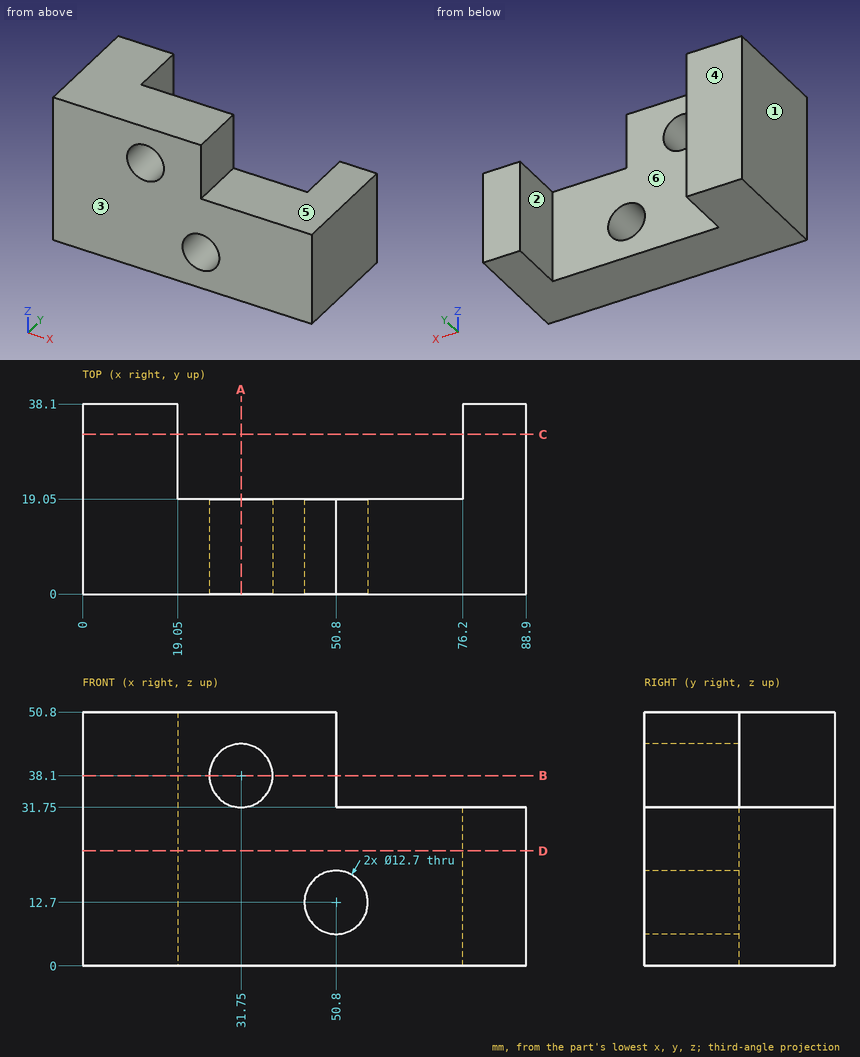
Geometry: see drawing. Coordinates: mm, zero at the bounding-box minimum. A direction names the side the tool comes from. Round coordinates to 2 decimals unless told otherwise and drop trailing zeros. Write each loop counter-clockwise with the first axis right and the second up, starting at its lowest first coordinate (ties: lowest second). Pieces come first, ordered by that corner, then holes.
1) Draft query along X for the marked faces 1, 2 and 3. Return one class per face: pulls with the +X half, pulls with the -X half, needs draft (parallel to the pull), parting line crosses it, or undercut.
2) Cut plane D-D (z = 23). Return the cut outline in (x, y), then the cut area to 3 significant figures.
3) Cut plane C-C (y = 32). Return the cut outline in (x, z).
4) Cut plane A-A (x = 31.75). Return the cut outline in (y, z), then the cut area to 3 significant figures.
5) Cut plane B-B (z = 38.1). Return the cut outline in (x, y).
6) Ray query, L1, parallel to X at y = 28, z = 2; L2, parallel to X at y = 11, z = 38.1; L3, parallel to Y at x = 43, z = 21.5. Return the intervals inside material, ascending.
7) Reachability of the marked faces 4, 5 and 6 from +Z, -Z, +X, -X, +Y, -Y: full face, straight path, thin tool, end or side. Return the list, or none.
8) Contact query for a flat-ended pin moving along its axis: P1, Ø15, axis at x = 51.5, z = 28.5, coming from the +Y side. Output: stop coordinate, or through.
Geometry says:
1. face 1: pulls with the -X half
1. face 2: undercut
1. face 3: needs draft
2. outline: (0, 0) - (88.9, 0) - (88.9, 38.1) - (76.2, 38.1) - (76.2, 19.05) - (19.05, 19.05) - (19.05, 38.1) - (0, 38.1) - close
2. area: 2,300 mm2
3. outline: (0, 0) - (19.05, 0) - (19.05, 50.8) - (0, 50.8) - close; (76.2, 0) - (88.9, 0) - (88.9, 31.75) - (76.2, 31.75) - close
4. outline: (0, 0) - (19.05, 0) - (19.05, 31.75) - (0, 31.75) - close; (0, 44.45) - (19.05, 44.45) - (19.05, 50.8) - (0, 50.8) - close
4. area: 726 mm2
5. outline: (0, 0) - (25.4, 0) - (25.4, 19.05) - (19.05, 19.05) - (19.05, 38.1) - (0, 38.1) - close; (38.1, 0) - (50.8, 0) - (50.8, 19.05) - (38.1, 19.05) - close
6. L1: x = 0 to 19.05, 76.2 to 88.9
6. L2: x = 0 to 25.4, 38.1 to 50.8
6. L3: y = 0 to 19.05
7. face 4: +Z, -Z, +X, -X, +Y
7. face 5: +Z, +X, +Y, -Y
7. face 6: +Z, -Z, +Y
8. P1: stops at y = 19.05
